Part model, mm, in its own coordinate system. Coordinates: 2 decimals unless noted, no trailing zeros. Write each loop counter-clockwise with the first axis right and the second up, starting at its lowest first coordinate (ties: lowest second). Pieces come first, ordered by that corner, then holes. Notation, with made-up numbers: M 7.25,57 L 51.25,57 A31 ccw 51.25,90 Z; hole C 67.25,-10.75 d9. An arc over 180 degrees is marked long. Use a Markdown table: item, result. Add a question column.
Q1. Mould opens along X. For faces 1 (the cylindrical face through (-17.137, -50.091, 58.177)), 2 (the flat face through (-19, -35, 54.74)), 3 (the flat face through (-19.491, -35.265, 58.684)), 4 (the flat face through (-22, -41, 53.74)) say: released by +X, released by -X, zero draft, split by the parting line, or undercut.
Q2. Pin check, flat tip, straight feed: pin 1 Ø4 at (y, z) = (-47.5, 61.5) entering from -X. Stop position of the tip, or through.
Q3. Slice it at B-B on x = -21.5. Write the cut outline in (y, z).
Q4. Slice it at C-C on z = 57.25. Write the cut outline in (x, y), then the cut area to 3 significant figures.
Q5. Slice it at A-A on y = -39.5. Write the cut outline in (x, z).
Q6. Wall check: L1, parallel to X at y = -36, z = 61.75; L2, parallel to X at y = -39.5, z = 55.5; L3, parallel to Y at x = -21.5, z = 57. Give the ranges that are in metal, low to high. Write a range as from..to.
Q7. Slice it at D-D on y = -47.75. Write the cut outline in (x, z).
from build123d import *

# Parameters (mm, degrees)
BOSS_EXTRUDE1_START = 53.740316
SKETCH1_R           = 9.85
BOSS_EXTRUDE1_DEPTH = 9
CUT_EXTRUDE1_START  = -9
SKETCH2_R           = 2.63
CUT_EXTRUDE1_DEPTH  = 1


with BuildPart() as part:
    # Sketch1 → Boss-Extrude1 (new body)
    with BuildSketch(Plane.XY.offset(BOSS_EXTRUDE1_START)):
        with Locations((-21.682123493, -41.352707657)):
            Circle(SKETCH1_R)
        with BuildLine():
            Line((-21.105209467, -34.677075087), (-17.830791495, -35.869629886))
            ThreePointArc((-17.830791495, -35.869629886), (-21.042183766, -39.595614277), (-21.105209467, -34.677075087))
        make_face(mode=Mode.SUBTRACT)
    extrude(amount=BOSS_EXTRUDE1_DEPTH)

    # Sketch2 → Cut-Extrude1 (cut)
    with BuildSketch(Plane.XY.offset(62.740315649).offset(CUT_EXTRUDE1_START)):
        with Locations((-20.142161583, -37.124408079)):
            Circle(SKETCH2_R)
    extrude(amount=CUT_EXTRUDE1_DEPTH, mode=Mode.SUBTRACT)


solid = part.part
Recorded:
| question | item | result |
|---|---|---|
| 1 | face 1 | split by the parting line |
| 1 | face 2 | undercut |
| 1 | face 3 | undercut |
| 1 | face 4 | zero draft |
| 2 | pin 1 | x = -30.62 |
| 3 | outline | M -51.2,53.74 L -39.38,53.74 L -39.38,62.74 L -51.2,62.74 Z; M -34.87,53.74 L -31.5,53.74 L -31.5,62.74 L -34.87,62.74 Z |
| 4 | outline | C -21.68,-41.35 d19.7; hole M -21.11,-34.68 A2.63 ccw long -17.83,-35.87 Z |
| 4 | area | 285 mm² |
| 5 | outline | M -31.36,53.74 L -21.27,53.74 L -21.27,62.74 L -31.36,62.74 Z; M -19.01,53.74 L -12.01,53.74 L -12.01,62.74 L -19.01,62.74 Z |
| 6 | L1 | -29.95..-22.52, -17.76..-13.41 |
| 6 | L2 | -31.36..-21.27, -19.01..-12.01 |
| 6 | L3 | -51.2..-39.38, -34.87..-31.5 |
| 7 | outline | M -29.17,53.74 L -14.19,53.74 L -14.19,62.74 L -29.17,62.74 Z |
